Here's how the part is built. I have some questions about the finished solid (model axes, mm). Face numbers are marked on the shaded views. A direction names the side the tool comes from. Give positions to 0.01 mm unless a question says otherwise; leave off trailing zeros. Loops run counter-clockwise (first coordinate to the right, second up) from the corner with the lowest first, then second, coordinate; pieces in that order, holes last. Notation, with made-up numbers: (52, 43.25) - (103, 43.25) arc R19 ccw to (103, 80.25) - close; hole circle Ø9 at (-15, -11.5). An arc over 180 degrees is marked (long way). Use a Markdown table: item, result.
from build123d import *
from OCP.BRepFilletAPI import BRepFilletAPI_MakeChamfer

# Parameters (mm, degrees)
SKETCH1_R                = 0.85
BOSS_EXTRUDE1_DEPTH      = 5
BOSS_EXTRUDE2_DEPTH      = 2
SKETCH3_R                = 2.25
BOSS_EXTRUDE3_DEPTH      = 5
SKETCH4_R                = 3.5
CUT_EXTRUDE1_DEPTH       = 3
SKETCH5_W                = 10
SKETCH5_H                = 10
CUT_EXTRUDE2_DEPTH       = 47.770717335
FILLET1_R                = 7
BOSS_EXTRUDE4_DEPTH      = 5
BOSS_EXTRUDE4_DEPTH_BACK = 8
SKETCH6_W                = 7.5
SKETCH6_H                = 20
SKETCH7_W                = 6
SKETCH7_H                = 9
BOSS_EXTRUDE5_DEPTH      = 27.5
SKETCH8_W                = 19.75
SKETCH8_H                = 9
BOSS_EXTRUDE6_DEPTH      = 7
SKETCH9_W                = 7.5
SKETCH9_H                = 5
BOSS_EXTRUDE7_DEPTH      = 11
CUT_EXTRUDE3_DEPTH       = 7.5
CHAMFER3_SIZE            = 0.5
CHAMFER1_SIZE            = 2.5
CHAMFER1_SIZE_2          = 1.25


with BuildPart() as part:
    # Sketch1 → Boss-Extrude1 (new body)
    with BuildSketch(Plane.XY):
        Polygon((-10, -35), (-10, 30), (10, 30), (10, -35), (17.5, -35), (17.5, 37.5), (-17.5, 37.5), (-17.5, -35), align=None)
        with Locations((-12.5, 32.5)):
            Circle(SKETCH1_R, mode=Mode.SUBTRACT)
        with Locations((12.5, 32.5)):
            Circle(SKETCH1_R, mode=Mode.SUBTRACT)
        with Locations((-12.5, -32.5)):
            Circle(SKETCH1_R, mode=Mode.SUBTRACT)
        with Locations((12.5, -32.5)):
            Circle(SKETCH1_R, mode=Mode.SUBTRACT)
    extrude(amount=BOSS_EXTRUDE1_DEPTH)

    # Sketch2 → Boss-Extrude2 (add)
    with BuildSketch(Plane.XY):
        Polygon((17.5, -35), (17.5, 37.5), (-17.5, 37.5), (-17.5, -35), (-15.1, -35), (-15.1, 35.1), (15.1, 35.1), (15.1, -35), align=None)
    extrude(amount=-BOSS_EXTRUDE2_DEPTH)

    # Sketch3 → Boss-Extrude3 (add)
    # profile 1 of 2: a face of its own
    with BuildSketch(Plane.XY):
        with BuildLine():
            Line((22.5, 5), (17.5, 5))
            Line((17.5, 5), (17.5, -5))
            Line((17.5, -5), (22.5, -5))
            ThreePointArc((22.5, -5), (27.5, 0), (22.5, 5))
        make_face()
        with Locations(Location((22.5, 0, 0), (0, 0, 180))):
            Circle(SKETCH3_R, mode=Mode.SUBTRACT)
    # profile 2 of 2: a face of its own
    with BuildSketch(Plane.XY):
        with BuildLine():
            Line((-22.5, 5), (-17.5, 5))
            Line((-17.5, 5), (-17.5, -5))
            Line((-17.5, -5), (-22.5, -5))
            ThreePointArc((-22.5, -5), (-27.5, 0), (-22.5, 5))
        make_face()
        with Locations(Location((-22.5, 0, 0), (0, 0, 180))):
            Circle(SKETCH3_R, mode=Mode.SUBTRACT)
    extrude(amount=BOSS_EXTRUDE3_DEPTH)

    # Sketch4 → Cut-Extrude1 (cut)
    with BuildSketch(Plane(origin=(0, 0, 0), x_dir=(-1, 0, 0), z_dir=(0, 0, -1))):
        with Locations((-22.5, 0)):
            Circle(SKETCH4_R)
        with Locations((22.5, 0)):
            Circle(SKETCH4_R)
    extrude(amount=-CUT_EXTRUDE1_DEPTH, mode=Mode.SUBTRACT)

    # Sketch5 → Cut-Extrude2 (cut, through all)
    with BuildSketch(Plane(origin=(0, 0, 0), x_dir=(-1, 0, 0), z_dir=(0, 0, -1))):
        with Locations((-12.5, 32.5)):
            Rectangle(SKETCH5_W, SKETCH5_H)
        with Locations((12.5, 32.5)):
            Rectangle(SKETCH5_W, SKETCH5_H)
    extrude(amount=CUT_EXTRUDE2_DEPTH, mode=Mode.SUBTRACT)

    # Fillet1
    fillet1_edges = [part.edges().sort_by_distance(p)[0] for p in [
        (-17.5, 37.5, 2.5),
        (17.5, 37.5, 2.5),
    ]]
    fillet(fillet1_edges, radius=FILLET1_R)

    # Sketch6 → Boss-Extrude4 (add, two sides: drawn at the far end of the back side and taken through both)
    with BuildSketch(Plane.XY.offset(-BOSS_EXTRUDE4_DEPTH_BACK)):
        with Locations((-13.75, -45)):
            Rectangle(SKETCH6_W, SKETCH6_H)
    extrude(amount=BOSS_EXTRUDE4_DEPTH + BOSS_EXTRUDE4_DEPTH_BACK)

    # Sketch7 → Boss-Extrude5 (add)
    with BuildSketch(Plane(origin=(-10, 0, 0), x_dir=(0, 0, -1), z_dir=(1, 0, 0))):
        with Locations((-2, -50.5)):
            Rectangle(SKETCH7_W, SKETCH7_H)
    extrude(amount=BOSS_EXTRUDE5_DEPTH)

    # Sketch8 → Boss-Extrude6 (add)
    with BuildSketch(Plane(origin=(0, 0, -1), x_dir=(-1, 0, 0), z_dir=(0, 0, -1))):
        with Locations((-7.625, -50.5)):
            Rectangle(SKETCH8_W, SKETCH8_H)
    extrude(amount=BOSS_EXTRUDE6_DEPTH)

    # Sketch9 → Boss-Extrude7 (add)
    with BuildSketch(Plane.XZ.offset(35)):
        with Locations((13.75, 2.5)):
            Rectangle(SKETCH9_W, SKETCH9_H)
    extrude(amount=BOSS_EXTRUDE7_DEPTH)

    # Sketch10 → Cut-Extrude3 (cut)
    with BuildSketch(Plane(origin=(17.5, 0, 0), x_dir=(0, 0, -1), z_dir=(1, 0, 0))):
        with BuildLine():
            Line((-4.5, -36.5), (-6, -36.5))
            Line((-6, -36.5), (-6, -44.5))
            Line((-6, -44.5), (-4.5, -44.5))
            ThreePointArc((-4.5, -44.5), (-3, -43), (-4.5, -41.5))
            Line((-4.5, -41.5), (-5, -41.5))
            Line((-5, -41.5), (-5, -39.5))
            Line((-5, -39.5), (-4.5, -39.5))
            ThreePointArc((-4.5, -39.5), (-3, -38), (-4.5, -36.5))
        make_face()
    extrude(amount=-CUT_EXTRUDE3_DEPTH, mode=Mode.SUBTRACT)

    # Chamfer3
    chamfer3_edges = [part.edges().sort_by_distance(p)[0] for p in [
        (0, 30, 5),
        (-17.5, 17.75, 5),
        (0, 37.5, 5),
        (15.449747468, 35.449747468, 5),
        (-15.449747468, 35.449747468, 5),
        (10, -3.25, 5),
        (0, -55, 5),
        (-10, -8, 5),
        (0, -46, 5),
        (-13.35, 32.5, 0),
        (-13.35, 32.5, 5),
        (10, -45.25, 5),
        (17.5, -20.75, 5),
        (13.75, -44.5, 5),
        (13.75, -36.5, 5),
        (17.5, -49.75, 5),
        (11.65, 32.5, 0),
        (11.65, 32.5, 5),
        (-13.35, -32.5, 0),
        (-13.35, -32.5, 5),
        (11.65, -32.5, 0),
        (11.65, -32.5, 5),
        (17.5, 17.75, 5),
        (27.5, 0, 5),
        (20, 5, 5),
        (20, -5, 5),
        (24.75, 0, 5),
        (-17.5, -30, 5),
        (-27.5, 0, 5),
        (-20, -5, 5),
        (-20, 5, 5),
        (-20.25, 0, 5),
    ]]
    chamfer(chamfer3_edges, length=CHAMFER3_SIZE - 0.0001)  # a hair under: the kernel refuses the full size

    # Chamfer1
    chamfer1_edges_1 = [part.edges().sort_by_distance(p)[0] for p in [
        (26, 0, 3),
    ]]
    chamfer1_side_1 = [part.faces().sort_by_distance(p)[0] for p in [
        (26, 0, 2.975),
    ]]
    chamfer1_edges_2 = [part.edges().sort_by_distance(p)[0] for p in [
        (-19, 0, 3),
    ]]
    chamfer1_side_2 = [part.faces().sort_by_distance(p)[0] for p in [
        (-19, 0, 2.975),
    ]]
    chamfer1 = BRepFilletAPI_MakeChamfer(part.part.solid().wrapped)
    for e in chamfer1_edges_1:
        chamfer1.Add(CHAMFER1_SIZE - 0.0001, CHAMFER1_SIZE_2 - 0.0001, e.wrapped, chamfer1_side_1[0].wrapped)
    for e in chamfer1_edges_2:
        chamfer1.Add(CHAMFER1_SIZE - 0.0001, CHAMFER1_SIZE_2 - 0.0001, e.wrapped, chamfer1_side_2[0].wrapped)
    add(Compound.cast(chamfer1.Shape()), mode=Mode.REPLACE)  # a hair under: the kernel refuses the full size


solid = part.part
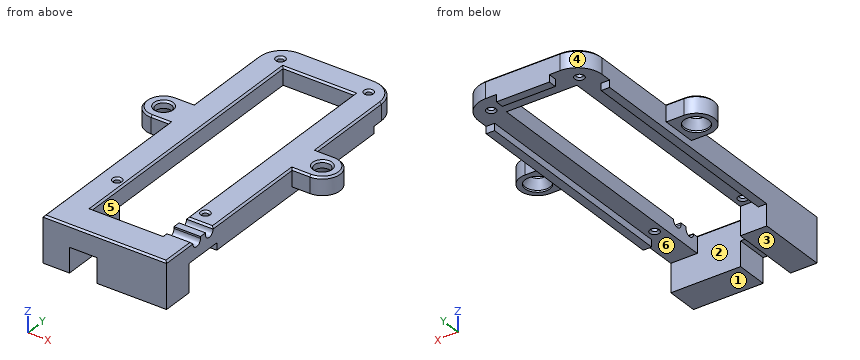
(1) If I drill on line 1 (X direction, y = -32.5, z = 1.9); line 2 (Y direction, x = -22.5, z = 0.3); line 3 (Y direction, x = 12.5, z = 1.45), over which ranges is the centre line in solid material (lowest first)?
A:
| item | result |
|---|---|
| line 1 | -17.5 to -13.35, -11.65 to -10, 10 to 11.65, 13.35 to 17.5 |
| line 2 | -5 to -3.5, 3.5 to 5 |
| line 3 | -55 to -33.35, -31.65 to 31.65, 33.35 to 37.21 |
(2) On a 3-axis mill with a long thin cutter (end or side, diameter ignored), from which of +Z, -Z, +X, -X, +Y, -Y can I reach the whole of each face in a straight line? I mean the marked faces 1 and 2. Say none if no direction works.
A:
| item | result |
|---|---|
| face 1 | -Z, +X, -X, +Y, -Y |
| face 2 | -Z |
(3) Suppose I cut it at C-C on y = -49. Write out the boundary of the cut face in (x, z), plus the area to 4 significant figures.
A:
| item | result |
|---|---|
| outline | (-17.5, -8) - (-10, -8) - (-10, -1) - (-2.25, -1) - (-2.25, -8) - (17.5, -8) - (17.5, 4.5) - (17, 5) - (-17, 5) - (-17.5, 4.5) - close |
| area | 400.5 mm2 |
(4) Suppose I cut it at B-B on z = -4.75. Write out the boundary of the cut face in (x, y).
A:
| item | result |
|---|---|
| outline | (-17.5, -55) - (-10, -55) - (-10, -35) - (-17.5, -35) - close; (-2.25, -55) - (17.5, -55) - (17.5, -46) - (-2.25, -46) - close |
(5) We'd pull the mould along X, two halves only. Please class the marked faces 3, 4, 5 and 6: pulls with the +X half, pulls with the -X half, needs draft (parallel to the pull), parting line crosses it, or undercut.
A:
| item | result |
|---|---|
| face 3 | needs draft |
| face 4 | pulls with the -X half |
| face 5 | undercut |
| face 6 | undercut |
(6) Suppose I cut it at A-A on y = -29.5. Write out the boundary of the cut face in (x, z).
A:
| item | result |
|---|---|
| outline | (-17.5, -2) - (-15.1, -2) - (-15.1, 0) - (-10, 0) - (-10, 4.5) - (-10.5, 5) - (-17, 5) - (-17.5, 4.5) - close; (10, 0) - (15.1, 0) - (15.1, -2) - (17.5, -2) - (17.5, 4.5) - (17, 5) - (10.5, 5) - (10, 4.5) - close |
(7) Will these pins go through, and if not, where does the flat tip stop? pin 1 (3.5 mm diameter, centred on x = -19, z = 1.5, fed in from -Y); pin 2 (1.6 mm diameter, centred on y = -13.5, z = -0.5, fed in from +X); pin 3 (2.5 mm diameter, centred on x = -16, y = -7.5, fed in from -Z); pin 4 (5 mm diameter, centred on y = -38, z = -6.5, fed in from +X).
A:
| item | result |
|---|---|
| pin 1 | y = -55 |
| pin 2 | x = 17.5 |
| pin 3 | z = -2 |
| pin 4 | x = -10 |
(8) Suppose I cut it at D-D on z = 2. Write out the boundary of the cut face in (x, y), plus the area to 3 significant figures.
A:
| item | result |
|---|---|
| outline | (-22.5, -5) - (-17.5, -5) - (-17.5, -55) - (17.5, -55) - (17.5, -5) - (22.5, -5) arc R5 ccw to (22.5, 5) - (17.5, 5) - (17.5, 30.5) arc R7 ccw to (10.5, 37.5) - (-10.5, 37.5) arc R7 ccw to (-17.5, 30.5) - (-17.5, 5) - (-22.5, 5) arc R5 ccw to start; hole circle Ø5.5 at (-22.5, 0); hole circle Ø1.7 at (-12.5, -32.5); hole circle Ø1.7 at (-12.5, 32.5); hole (-10, -46) - (10, -46) - (10, 30) - (-10, 30) - close; hole circle Ø1.7 at (12.5, -32.5); hole circle Ø1.7 at (12.5, 32.5); hole circle Ø5.5 at (22.5, 0) |
| area | 1,820 mm2 |
